The drawing under review shows one solid part. Ordinate dimensions are in mm from its lowest x, y, z. Give positions to 0.01 mm unless a question says otherwise; leave off trailing zeros. Write each loop counter-clockwise with the first axis right and the second up, starting at its lowest first coordinate (ties: lowest second). Pieces come first, ordered by that corner, then holes. Notation, with made-up numbers: (38.25, -23.75) -> (93.25, -23.75) arc R13 cw to (93.25, -6.75) -> close; hole circle Ø8 at (44, 75.5). An arc over 180 degrees is marked (long way). Use CSV: the item, a comma, the result in double quotes.
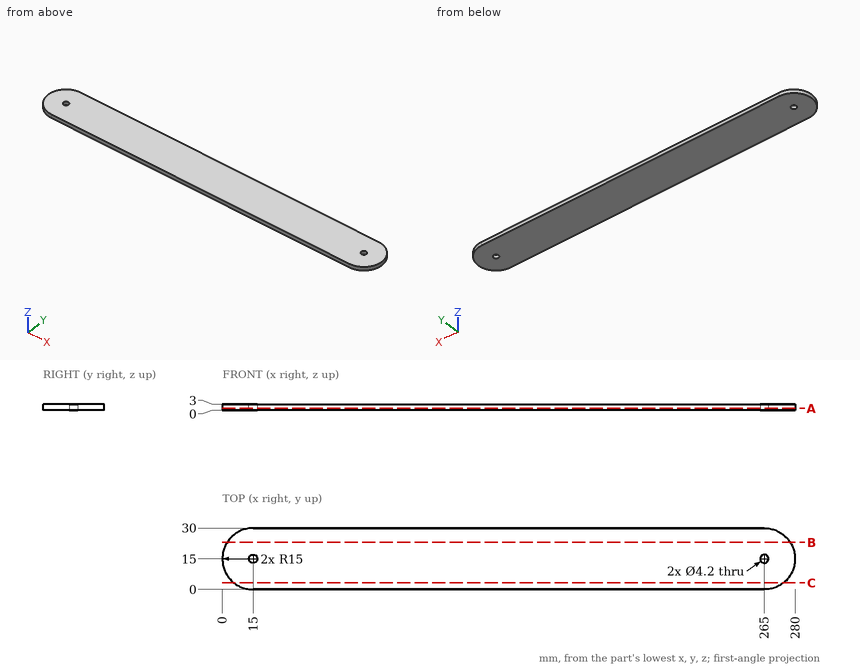
(1) For line 1 along X through (y, z) = (15.25, 2.15); line 2 along Y through (x, z) = (265, 0.8); line 3 along X through (y, z) = (15.5, 1.6), list the stretches that pass through material, from the lowest coordinate up. Write a range as [from, to].
Established:
line 1,"x = [0, 12.91], [17.09, 262.91], [267.09, 280]"
line 2,"y = [0, 12.9], [17.1, 30]"
line 3,"x = [0.01, 12.96], [17.04, 262.96], [267.04, 279.99]"
(2) Take a section at B-B (y = 23). Write out the cut boundary in (x, z).
Established:
outline,"(2.31, 0) -> (277.69, 0) -> (277.69, 3) -> (2.31, 3) -> close"
(3) Take a section at C-C (y = 3.25). Write out the cut boundary in (x, z), then the cut area to 3 significant figures.
Established:
outline,"(5.68, 0) -> (274.32, 0) -> (274.32, 3) -> (5.68, 3) -> close"
area,"806 mm2"
(4) Take a section at A-A (z = 0.8). Write out the cut boundary in (x, y), then the cut area to 3 significant figures.
Established:
outline,"(15, 0) -> (265, 0) arc R15 ccw to (265, 30) -> (15, 30) arc R15 ccw to start; hole circle Ø4.2 at (15, 15); hole circle Ø4.2 at (265, 15)"
area,"8,180 mm2"
